Part model, mm, in its own coordinate system. Face numbers are marked on the shaded views. A direction names the side the tool comes from. Round coordinates to 2 decimals unless told otherwise and drop trailing zeros. Loops run counter-clockwise (first coordinate to the right, second up) from the corner with the lowest first, then second, coordinate; pieces in that order, holes last. Notation, with made-up numbers: M -19,86 L 36,86 A28 ccw 36,124 Z; hole C -28.75,34.5 d5. An arc over 180 degrees is marked long. Answer as CSV lines item,"result". Start each with the question number.
Item 1: Mould opens along Y. For the marked faces 1, 2 and 3 say: pulls with the +Y half, pulls with the -Y half, needs draft (parallel to the pull), parting line crosses it, or undercut.
Item 2: Band-saw the part on C-C (x = 3.3). Give the cut face in (y, z).
Item 3: Wall check: line 1 (Y direction, x = 0.25, z = 0); line 2 (Y direction, x = 0.1, z = 0); line 3 (X direction, y = 3.25, z = -0.5). Give the ranges that are in metal, low to high.
Item 4: Which spindle directions (+Z, -Z, +X, -X, +Y, -Y) get a long thin tool onto all of the face, cutting with end or side? Do the marked faces 4 and 5. Say none if no direction does.
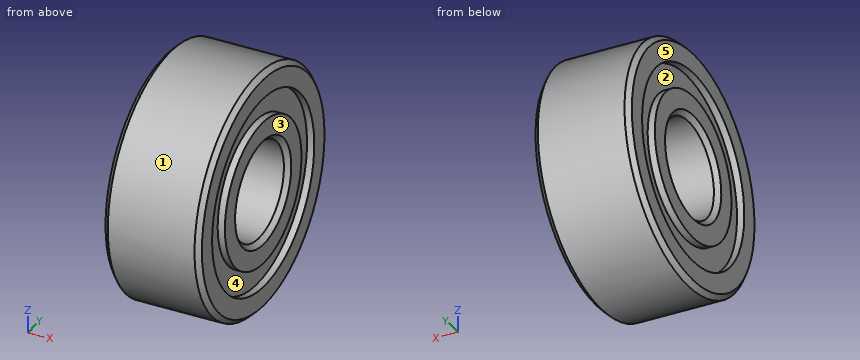
```python
from build123d import *

# Parameters (mm, degrees)
SKETCH_1_R          = 5
SKETCH_1_R_2        = 2
EXTRUDE_1_DEPTH     = 4
SKETCH_2_R          = 4
SKETCH_2_R_2        = 3
CUT_EXTRUDE_1_DEPTH = 0.3
CHAMFER_1_SIZE      = 0.2
SKETCH_3_R          = 4
SKETCH_3_R_2        = 3
CUT_EXTRUDE_2_DEPTH = 0.3


with BuildPart() as part:
    # 草图1 → 凸台-拉伸1 (new body)
    with BuildSketch(Plane(origin=(0, 0, 0), x_dir=(0, 0, -1), z_dir=(1, 0, 0))):
        Circle(SKETCH_1_R)
        Circle(SKETCH_1_R_2, mode=Mode.SUBTRACT)
    extrude(amount=EXTRUDE_1_DEPTH)

    # 草图2 → 切除-拉伸1 (cut)
    with BuildSketch(Plane(origin=(4, 0, 0), x_dir=(0, 0, -1), z_dir=(1, 0, 0))):
        with Locations((-0.000375625, 0)):
            Circle(SKETCH_2_R)
        with Locations((-0.000375625, 0)):
            Circle(SKETCH_2_R_2, mode=Mode.SUBTRACT)
    extrude(amount=-CUT_EXTRUDE_1_DEPTH, mode=Mode.SUBTRACT)

    # 倒角1
    chamfer_1_edges = [part.edges().sort_by_distance(p)[0] for p in [
        (0, 0, 5),
        (4, 0, 5),
        (0, 0, 2),
        (4, 0, 2),
    ]]
    chamfer(chamfer_1_edges, length=CHAMFER_1_SIZE)

    # 草图3 → 切除-拉伸2 (cut)
    with BuildSketch(Plane.ZY):
        Circle(SKETCH_3_R)
        Circle(SKETCH_3_R_2, mode=Mode.SUBTRACT)
    extrude(amount=-CUT_EXTRUDE_2_DEPTH, mode=Mode.SUBTRACT)


solid = part.part
```
Answer block:
1,face 1,"parting line crosses it"
1,face 2,"undercut"
1,face 3,"needs draft"
2,outline,"C 0,0 d10; hole C 0,0 d4"
3,line 1,"y = -5 to -4, -3 to -2, 2 to 3, 4 to 5"
3,line 2,"y = -4.9 to -4, -3 to -2.1, 2.1 to 3, 4 to 4.9"
3,line 3,"x = 0.3 to 3.7"
4,face 4,"+X"
4,face 5,"+Z, -Z, -X, +Y, -Y"
